```python
from build123d import *

# Parameters (mm, degrees)
BOSS_EXTRUDE1_DEPTH     = 501.65
SKETCH2_R               = 1.984375
CUT_EXTRUDE1_DEPTH      = 502.8276078
SKETCH3_R               = 1.984375
CUT_EXTRUDE2_DEPTH      = 502.8276078
CUT_EXTRUDE4_DEPTH      = 502.8276078
CUT_EXTRUDE4_DEPTH_BACK = 502.8276078
SKETCH4_R               = 3.175


with BuildPart() as part:
    # Sketch1 → Boss-Extrude1 (new body)
    with BuildSketch(Plane.XY):
        Polygon((0, 0), (-8.980256121, 8.980256121), (-9.878281733, 8.082230509), (0, -1.796051224), (9.878281733, 8.082230509), (8.980256121, 8.980256121), align=None)
    extrude(amount=BOSS_EXTRUDE1_DEPTH)

    # Sketch2 → Cut-Extrude1 (cut, through all)
    with BuildSketch(Plane(origin=(0, 0, 0), x_dir=(0, 0, 1), z_dir=(-0.7071067811865471, 0.7071067811865479, 0))):
        with Locations(Location((6.35, 7.62, 0), (0, 0, 270))):
            Circle(SKETCH2_R)
        with Locations(Location((19.05, 7.62, 0), (0, 0, 270))):
            Circle(SKETCH2_R)
    extrude(amount=-CUT_EXTRUDE1_DEPTH, mode=Mode.SUBTRACT)

    # Sketch3 → Cut-Extrude2 (cut, through all)
    with BuildSketch(Plane(origin=(0, 0, 0), x_dir=(0, 0, -1), z_dir=(0.7071067811865482, 0.7071067811865468, 0))):
        with Locations(Location((-12.7, 7.62, 0), (0, 0, 90))):
            Circle(SKETCH3_R)
    extrude(amount=-CUT_EXTRUDE2_DEPTH, mode=Mode.SUBTRACT)

    # Sketch4 → Cut-Extrude4 (cut, two sides: drawn at the far end of the back side and taken through both)
    with BuildSketch(Plane(origin=(0, 0, 0), x_dir=(1, 0, 0), z_dir=(0, 1, 0)).offset(-CUT_EXTRUDE4_DEPTH_BACK)):
        with Locations(Location((0, -438.15, 0), (0, 0, 270))):
            Circle(SKETCH4_R)
        with Locations(Location((0, -361.95, 0), (0, 0, 270))):
            Circle(SKETCH4_R)
    extrude(amount=CUT_EXTRUDE4_DEPTH + CUT_EXTRUDE4_DEPTH_BACK, mode=Mode.SUBTRACT)


solid = part.part
```
Model file for the job. Use its own axes, mm. A direction names the side the tool comes from. Coordinates: 2 decimals unless noted, no trailing zeros. Loops run counter-clockwise (first coordinate to the right, second up) from the corner with the lowest first, then second, coordinate; pieces in that order, holes last. Notation, with made-up numbers: (5.5, 88.5) -> (44.5, 88.5) arc R21 ccw to (44.5, 95.5) -> close; hole circle Ø4 at (76, 53.25). An arc over 180 degrees is marked (long way). Answer as a JSON object with one key per item and string values.
Q1. Probe probe 1 along Z at (x, y) = (0, -0.05) (3 decimals); probe 2 along X at (y, z) = (8.25, 214); probe 3 along X at (y, z) = (7, 42). List the from-to ranges inside material, lowest first.
Report:
{"probe 1": "z = 0 to 358.775, 365.125 to 434.975, 441.325 to 501.65", "probe 2": "x = -9.71 to -8.25, 8.25 to 9.71", "probe 3": "x = -8.8 to -7, 7 to 8.8"}
Q2. Pull direction X, two halves, no side cores. Call faces 1 (the flat face through (-4, 4, 247)), 2 (the flat face through (4.87, 3.074, 247.313)), 3 (the flat face through (-2.24, 2.02, 501.65)): released by +X, released by -X, zero draft, split by the parting line, or undercut.
Report:
{"face 1": "undercut", "face 2": "released by +X", "face 3": "zero draft"}
Q3. 3-axis set-ups, long thin cutter, end or side, ignore diameter. For faces 4 (the flat face through (-5.008, 3.212, 247.313)), 5 (the flat face through (5, 5, 247)): which of +Z, -Z, +X, -X, +Y, -Y reach the whole face in a straight line?
Report:
{"face 4": "+Z, -Z, -X, -Y", "face 5": "+Z, -Z, +Y"}
Q4. Flat gauge pins, fed straight in: P1, Ø3, axis at y = 1.5, z = 239.5, coming from the -X side; P2, Ø1, axis at x = -5.5, z = 105.5, coming from the -Y side; P3, Ø1.5, axis at x = -7.5, z = 323.5, coming from the +Y side. Where does each tip first touch, or does it go through?
Report:
{"P1": "stops at x = -4.8", "P2": "stops at y = 3.2", "P3": "stops at y = 8.25"}
Q5. Cut at A-A (z = 343.5). List the corners of the cut face in (x, y), and give its area (3 significant figures).
Report:
{"outline": "(-9.88, 8.08) -> (0, -1.8) -> (9.88, 8.08) -> (8.98, 8.98) -> (0, 0) -> (-8.98, 8.98) -> close", "area": "33.9 mm2"}
